Drawing for the job (mm, zero at the part's lowest x, y, z). Round coordinates to 2 decimals unless told otherwise and drop trailing zeros. Order: outer loops, then holes, each group sorted by start corner. A loop starts at its lowest first (then second) coordinate and runs counter-clockwise, first axis right, second up. Notation, with made-up numbers: M 2.25,8 L 16.25,8 A17 ccw 16.25,36 Z; hole C -14,1 d6. An arc over 180 degrees is marked long. One line per item, written item: value. Start each with the question number.
Item 1: Band-saw the part on B-B, the plane y = 26.5. Write the cut outline in (x, z).
Item 2: Band-saw the part on A-A, the plane z = 3.5. Write the cut outline in (x, y).
Item 3: Pin check, flat tips, straight feed: pin 1 (1.5 mm diameter, centred on y = 1.5, z = 2.5, fed in from +X); pin 2 (1 mm diameter, centred on x = 69, y = 7.5, fed in from -Z); pin 3 (1.2 mm diameter, centred on x = 2.5, z = 2, fed in from +Y); pin 4 (1.2 mm diameter, centred on x = 3.5, z = 3, fed in from -Y). Stop position of each tip, or through.
Item 4: Probe L1, parallel to X at y = 27.5, z = 2.8. List the from-to ranges inside material, lowest first.
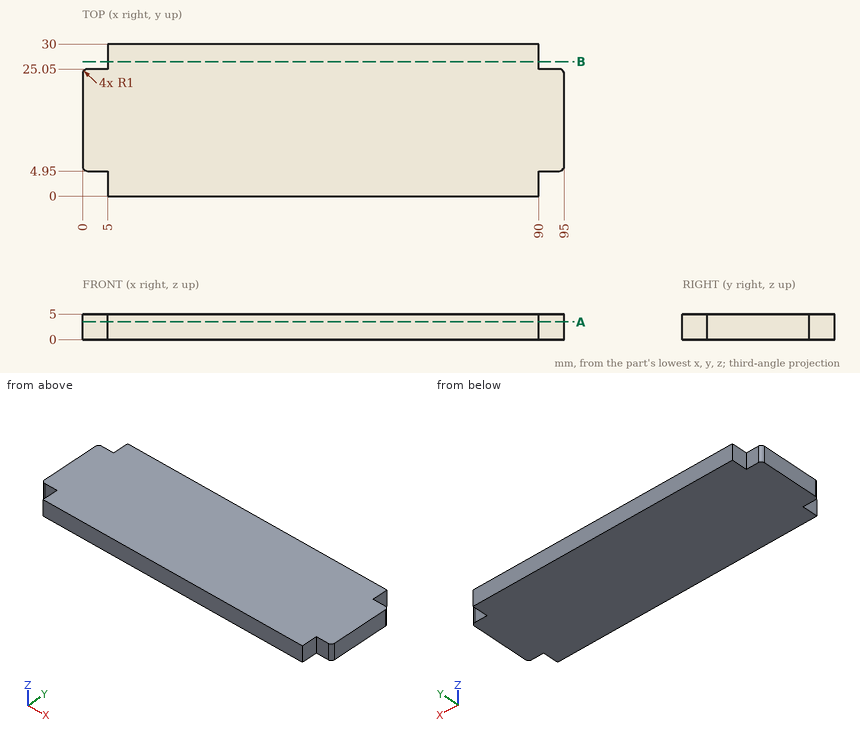
Output:
1. outline: M 5,0 L 90,0 L 90,5 L 5,5 Z
2. outline: M 0,5.95 A1 ccw 1,4.95 L 5,4.95 L 5,0 L 90,0 L 90,4.95 L 94,4.95 A1 ccw 95,5.95 L 95,24.05 A1 ccw 94,25.05 L 90,25.05 L 90,30 L 5,30 L 5,25.05 L 1,25.05 A1 ccw 0,24.05 Z
3. pin 1: stops at x = 90
3. pin 2: stops at z = 0
3. pin 3: stops at y = 25.05
3. pin 4: stops at y = 4.95
4. L1: x = 5 to 90
